Verification items for the finished model (mm, model axes). A direction names the side the tool comes from. Round coordinates to 2 decimals unless told otherwise and drop trailing zeros. Write each loop counter-clockwise with the first axis right and the second up, starting at its lowest first coordinate (ties: lowest second). Pieces come first, ordered by that corner, then holes. Notation, with made-up numbers: (22.5, 68) - (67.5, 68) arc R21 cw to (67.5, 84) - close; hole circle Ø1 at (75, 74). An arc over 180 degrees is marked (long way). Answer as a JSON object with one key per item and string values. Group by question number.
1) Mould release check, pull along X, two halves, no side actions. Record for faces 1 (the flat face through (-8, 3.175, 72)), 2 (the flat face through (-9, 0, 72)), 3 (the cylindrical face through (123.187, 2.817, -50.236)), 4 (the cylindrical face through (122.387, 2.898, -0.332)): +X half, -X half, draft (parallel to the pull), parting line (faces both ways), or undercut.
2) Section check D-D (z = 0). Enter the section's corners in (x, y) (3 decimals).
3) Section check A-A (z = 40). Enter the section's corners in (x, y) (3 decimals), then the cut area to 3 significant figures.
4) Set-up check for faces 5 (the flat face through (2, 3, 81.756)), 6 (the flat face through (115, 2, -51.594)): record each of +Z, -Z, +X, -X, +Y, -Y from which the full face is reachable in a straight line by a thin tool's end or side.
5) Section check C-C (y = 4.75). Enter the section's corners in (x, z) (1 decimal), then the cut area to 3 significant figures.
6) Go/stop test with flat-tipped pins: pin 1 Ø2 at (x, y) = (18.5, 4.5) entering from -Z; pin 2 Ø6 at (x, z) = (-119.86, 0) entering from -Y; pin 3 Ø2.5 at (x, y) = (-22, 1) entering from -Z. Record where each tip stops, or that it passes through.
7) Thickness scan on line 1 (X direction, y = 4.65, z = 0); line 2 (Z direction, x = -111, y = 5.35); line 3 (X direction, y = 1.6, z = 4). Record the ranges inside material, lowest first.
8) Section check B-B (x = -77). Enter the section's corners in (y, z) (3 decimals).
```python
from build123d import *

# Parameters (mm, degrees)
BOSS_EXTRUDE1_DEPTH = 3.175
BOSS_EXTRUDE2_DEPTH = 2.54
SKETCH3_R           = 2.5527
CUT_EXTRUDE1_DEPTH  = 153.360472739


with BuildPart() as part:
    # Sketch1 → Boss-Extrude1 (new body)
    with BuildSketch(Plane(origin=(0, 0, 0), x_dir=(1, 0, 0), z_dir=(0, 1, 0))):
        with BuildLine():
            Line((-64.29375, 80.16875), (-64.29375, 69.05625))
            Line((-64.29375, 69.05625), (-108.74375, 69.05625))
            Line((-108.74375, 69.05625), (-108.74375, -69.05625))
            Line((-108.74375, -69.05625), (108.74375, -69.05625))
            Line((108.74375, -69.05625), (108.74375, 51.59375))
            Line((108.74375, 51.59375), (119.85625, 51.59375))
            ThreePointArc((119.85625, 51.59375), (123.223846045, 50.198846045), (124.61875, 46.83125))
            Line((124.61875, 46.83125), (124.61875, -76.99375))
            ThreePointArc((124.61875, -76.99375), (123.223846045, -80.361346045), (119.85625, -81.75625))
            Line((119.85625, -81.75625), (-119.85625, -81.75625))
            ThreePointArc((-119.85625, -81.75625), (-123.223846045, -80.361346045), (-124.61875, -76.99375))
            Line((-124.61875, -76.99375), (-124.61875, 80.16875))
            ThreePointArc((-124.61875, 80.16875), (-123.223846045, 83.536346045), (-119.85625, 84.93125))
            Line((-119.85625, 84.93125), (-69.05625, 84.93125))
            ThreePointArc((-69.05625, 84.93125), (-65.688653955, 83.536346045), (-64.29375, 80.16875))
        make_face()
    extrude(amount=BOSS_EXTRUDE1_DEPTH)

    # Sketch2 → Boss-Extrude2 (add)
    with BuildSketch(Plane(origin=(0, 3.175, 0), x_dir=(1, 0, 0), z_dir=(0, 1, 0))):
        with BuildLine():
            Line((-64.29375, 80.16875), (-64.29375, 75.40625))
            Line((-64.29375, 75.40625), (-115.09375, 75.40625))
            Line((-115.09375, 75.40625), (-115.09375, -75.40625))
            Line((-115.09375, -75.40625), (115.09375, -75.40625))
            Line((115.09375, -75.40625), (115.09375, 51.59375))
            Line((115.09375, 51.59375), (119.85625, 51.59375))
            ThreePointArc((119.85625, 51.59375), (123.223846045, 50.198846045), (124.61875, 46.83125))
            Line((124.61875, 46.83125), (124.61875, -76.99375))
            ThreePointArc((124.61875, -76.99375), (123.223846045, -80.361346045), (119.85625, -81.75625))
            Line((119.85625, -81.75625), (-119.85625, -81.75625))
            ThreePointArc((-119.85625, -81.75625), (-123.223846045, -80.361346045), (-124.61875, -76.99375))
            Line((-124.61875, -76.99375), (-124.61875, 80.16875))
            ThreePointArc((-124.61875, 80.16875), (-123.223846045, 83.536346045), (-119.85625, 84.93125))
            Line((-119.85625, 84.93125), (-69.05625, 84.93125))
            ThreePointArc((-69.05625, 84.93125), (-65.688653955, 83.536346045), (-64.29375, 80.16875))
        make_face()
    extrude(amount=BOSS_EXTRUDE2_DEPTH)

    # Sketch3 → Cut-Extrude1 (cut, through all)
    with BuildSketch(Plane(origin=(0, 5.715, -5.715), x_dir=(-1, 0, 0), z_dir=(0, 1, 0))):
        with Locations(Location((119.85625, -63.34125, 0), (0, 0, 90))):
            Circle(SKETCH3_R)
        with Locations(Location((119.85625, 74.77125, 0), (0, 0, 90))):
            Circle(SKETCH3_R)
        with Locations(Location((119.85625, 5.715, 0), (0, 0, 90))):
            Circle(SKETCH3_R)
        with Locations(Location((-119.85625, 74.77125, 0), (0, 0, 90))):
            Circle(SKETCH3_R)
        with Locations(Location((-119.85625, 5.715, 0), (0, 0, 90))):
            Circle(SKETCH3_R)
    extrude(amount=-CUT_EXTRUDE1_DEPTH, mode=Mode.SUBTRACT)


solid = part.part
```
Returned:
{
 "1": {"face 1": "undercut", "face 2": "draft", "face 3": "+X half", "face 4": "undercut"},
 "2": {"outline": "(-124.619, 0) - (-122.409, 0) - (-122.409, 5.715) - (-124.619, 5.715) - close; (-117.304, 0) - (-108.744, 0) - (-108.744, 3.175) - (-115.094, 3.175) - (-115.094, 5.715) - (-117.304, 5.715) - close; (108.744, 0) - (117.304, 0) - (117.304, 5.715) - (115.094, 5.715) - (115.094, 3.175) - (108.744, 3.175) - close; (122.409, 0) - (124.619, 0) - (124.619, 5.715) - (122.409, 5.715) - close"},
 "3": {"outline": "(-124.619, 0) - (-108.744, 0) - (-108.744, 3.175) - (-115.094, 3.175) - (-115.094, 5.715) - (-124.619, 5.715) - close; (108.744, 0) - (124.619, 0) - (124.619, 5.715) - (115.094, 5.715) - (115.094, 3.175) - (108.744, 3.175) - close", "area": "149 mm2"},
 "4": {"face 5": "+Z, +X, -X, +Y, -Y", "face 6": "-Z, +X, +Y, -Y"},
 "5": {"outline": "(-124.6, -80.2) arc R4.8 ccw to (-119.9, -84.9) - (-69.1, -84.9) arc R4.8 ccw to (-64.3, -80.2) - (-64.3, -75.4) - (-115.1, -75.4) - (-115.1, 75.4) - (115.1, 75.4) - (115.1, -51.6) - (119.9, -51.6) arc R4.8 ccw to (124.6, -46.8) - (124.6, 77) arc R4.8 ccw to (119.9, 81.8) - (-119.9, 81.8) arc R4.8 ccw to (-124.6, 77) - close; hole circle Ø5.1 at (-119.9, -69.1); hole circle Ø5.1 at (-119.9, 0); hole circle Ø5.1 at (-119.9, 69.1); hole circle Ø5.1 at (119.9, 0); hole circle Ø5.1 at (119.9, 69.1)", "area": "4,680 mm2"},
 "6": {"pin 1": "z = 75.41", "pin 2": "y = 0", "pin 3": "z = 69.06"},
 "7": {"line 1": "-124.62 to -122.41, -117.3 to -115.09, 115.09 to 117.3, 122.41 to 124.62", "line 2": "-84.93 to -75.41, 75.41 to 81.76", "line 3": "-124.62 to -108.74, 108.74 to 124.62"},
 "8": {"outline": "(0, -84.931) - (5.715, -84.931) - (5.715, -75.406) - (3.175, -75.406) - (3.175, -69.056) - (0, -69.056) - close; (0, 69.056) - (3.175, 69.056) - (3.175, 75.406) - (5.715, 75.406) - (5.715, 81.756) - (0, 81.756) - close"}
}
